Read the model definition and answer for the solid it produces. Units are mm, in the model's axes. A direction names the side the tool comes from. Coordinates: 2 decimals unless noted, no trailing zeros. Order: outer loops, then holes, each group sorted by start corner. A loop starts at its lowest first (then second) coordinate and runs counter-clockwise, first axis right, second up. Notation, with made-up numbers: (62.25, 24) -> (109.25, 24) arc R4 ccw to (109.25, 29) -> close; hole circle Ø3 at (52, 72). An arc over 180 degrees is marked (long way). Return JSON: item names as keys, results as strings. Group by question number.
```python
from build123d import *

# Parameters (mm, degrees)
F0_W     = 94.996
F0_H     = 79.756
F0_W_2   = 10.16
F0_H_2   = 7.62
F1_DEPTH = 5.08
F2_W     = 70.612
F2_H     = 54.61
F3_DEPTH = 1.524
F5_DEPTH = 25.4
F6_R     = 1.905
F7_DEPTH = 25.4
F8_W     = 24.773464
F8_H     = 13.97
F9_DEPTH = 3.81


with BuildPart() as f1:
    # F0 (on Top) → F1 (new body)
    with BuildSketch(Plane.XY):
        with Locations((47.498, 39.878)):
            Rectangle(F0_W, F0_H)
        with Locations((19.304, 18.034)):
            Rectangle(F0_W_2, F0_H_2, mode=Mode.SUBTRACT)
        Polygon((14.224, 65.532), (80.772, 65.532), (80.772, 14.224), (29.464, 14.224), (29.464, 34.544), (14.224, 34.544), align=None, mode=Mode.SUBTRACT)
    extrude(amount=F1_DEPTH)

    # F2 (on face) → F3 (cut)
    with BuildSketch(Plane(origin=(0, 0, 0), x_dir=(1, 0, 0), z_dir=(0, 0, -1))):
        with Locations((48.006, -41.529)):
            Rectangle(F2_W, F2_H)
    extrude(amount=-F3_DEPTH, mode=Mode.SUBTRACT)

    # F4 (on face) → F5 (cut)
    with BuildSketch(Plane(origin=(0, 0, 1.524), x_dir=(1, 0, 0), z_dir=(0, 0, -1))):
        with BuildLine():
            Line((80.772, -32.258), (80.772, -35.80123))
            ThreePointArc((80.772, -35.80123), (82.399452, -34.029615), (80.772, -32.258))
        make_face()
    extrude(amount=-F5_DEPTH, mode=Mode.SUBTRACT)

    # F6 (on face) → F7 (cut)
    with BuildSketch(Plane(origin=(0, 0, 0), x_dir=(1, 0, 0), z_dir=(0, 0, -1))):
        with Locations((6.35, -8.077516)):
            Circle(F6_R)
        with Locations((88.138, -8.077516)):
            Circle(F6_R)
        with Locations((6.35, -74.117516)):
            Circle(F6_R)
        with Locations((88.138, -74.117516)):
            Circle(F6_R)
    extrude(amount=-F7_DEPTH, mode=Mode.SUBTRACT)

    # F8 (on face) → F9 (cut)
    with BuildSketch(Plane.XY.offset(5.08)):
        with Locations((8.389047, 46.101)):
            Rectangle(F8_W, F8_H)
    extrude(amount=-F9_DEPTH, mode=Mode.SUBTRACT)


solid = f1.part
```
1. For a pull along Y with two mould halves and no side action, classify faces 4 (the face through (0, 39, 1)), 5 (the face through (22, 34.544, 3)), 6 (the face through (47, 0, 3)) as released by +Y, released by -Y, zero draft, split by the parting line, or undercut.
2. Find section C-C on x = 45.5. Determine the outline of the cut face in (y, z), and give its area (3 significant figures).
3. Given pin 1 (8.5 mm diameter, centred on x = 17.5, y = 31.5, fed in from -Z), flat-ended and moving along its own axis, determine where the tip first touches the part or whether it passes through.
4. Find section D-D on z = 3.5. Determine the outline of the cut face in (x, y) (3 decimals), and give its area (3 significant figures).
5. Which of the six approach directions +Z, -Z, +X, -X, +Y, -Y give full straight-line access (tool end or side, diameter ignored) to faces 1 (the face through (7, 53.086, 3)), 2 (the face through (47, 14, 0)), 3 (the face through (80.772, 51, 3))?
6. Find section B-B on x = 6.35. Determine the outline of the cut face in (y, z).
7. Find section A-A on y = 26. Determine the outline of the cut face in (x, z).
8. Straight lines are drawn through the part: L1, parallel to X at y = 74, z = 4.1; L2, parallel to Y at x = 6.35, z = 2.9; L3, parallel to X at y = 19, z = 4.5. For each, find the intervals that lie inside material, in ascending order.
Result:
{
 "1": {"face 4": "zero draft", "face 5": "undercut", "face 6": "released by -Y"},
 "2": {"outline": "(0, 0) -> (14.22, 0) -> (14.22, 5.08) -> (0, 5.08) -> close; (65.53, 1.52) -> (68.83, 1.52) -> (68.83, 0) -> (79.76, 0) -> (79.76, 5.08) -> (65.53, 5.08) -> close", "area": "139 mm^2"},
 "3": {"pin 1": "z = 1.52"},
 "4": {"outline": "(0, 0) -> (94.996, 0) -> (94.996, 79.756) -> (0, 79.756) -> (0, 53.086) -> (14.224, 53.086) -> (14.224, 65.532) -> (80.772, 65.532) -> (80.772, 35.801) arc R1.778 cw to (80.772, 32.258) -> (80.772, 14.224) -> (29.464, 14.224) -> (29.464, 34.544) -> (14.224, 34.544) -> (14.224, 39.116) -> (0, 39.116) -> close; hole circle Ø3.81 at (6.35, 8.078); hole circle Ø3.81 at (6.35, 74.118); hole (14.224, 14.224) -> (24.384, 14.224) -> (24.384, 21.844) -> (14.224, 21.844) -> close; hole circle Ø3.81 at (88.138, 8.078); hole circle Ø3.81 at (88.138, 74.118)", "area": "4,150 mm^2"},
 "5": {"face 1": "+Z, -X", "face 2": "-Z, +X, -X, +Y, -Y", "face 3": "+Z, -Z"},
 "6": {"outline": "(0, 0) -> (6.17, 0) -> (6.17, 5.08) -> (0, 5.08) -> close; (9.98, 0) -> (72.21, 0) -> (72.21, 5.08) -> (53.09, 5.08) -> (53.09, 1.27) -> (39.12, 1.27) -> (39.12, 5.08) -> (9.98, 5.08) -> close; (76.02, 0) -> (79.76, 0) -> (79.76, 5.08) -> (76.02, 5.08) -> close"},
 "7": {"outline": "(0, 0) -> (12.7, 0) -> (12.7, 1.52) -> (29.46, 1.52) -> (29.46, 5.08) -> (0, 5.08) -> close; (80.77, 1.52) -> (83.31, 1.52) -> (83.31, 0) -> (95, 0) -> (95, 5.08) -> (80.77, 5.08) -> close"},
 "8": {"L1": "0 to 4.45, 8.25 to 86.24, 90.04 to 95", "L2": "0 to 6.17, 9.98 to 39.12, 53.09 to 72.21, 76.02 to 79.76", "L3": "0 to 14.22, 24.38 to 29.46, 80.77 to 95"}
}
